from build123d import *

# Parameters (mm, degrees)
SKETCH1_W                = 19
SKETCH1_H                = 19
BOSS_EXTRUDE1_DEPTH      = 1.5
SKETCH2_W                = 5
SKETCH2_H                = 5
CUT_EXTRUDE1_DEPTH       = 30.054329533
BOSS_EXTRUDE2_DEPTH      = 10
BOSS_EXTRUDE2_DEPTH_BACK = 1.5
SKETCH4_W                = 1
SKETCH4_H                = 19
SKETCH5_W                = 21
SKETCH5_H                = 1
BOSS_EXTRUDE3_DEPTH      = 19
SKETCH6_W                = 5
SKETCH6_H                = 5
CUT_EXTRUDE2_DEPTH       = 33.074717791
SKETCH7_W                = 3.862532253
SKETCH7_H                = 19
CUT_EXTRUDE3_DEPTH       = 1


with BuildPart() as part:
    # Sketch1 → Boss-Extrude1 (new body)
    with BuildSketch(Plane.XY):
        with Locations((-17.316728365, -1.580033592)):
            Rectangle(SKETCH1_W, SKETCH1_H)
    extrude(amount=BOSS_EXTRUDE1_DEPTH)

    # Sketch2 → Cut-Extrude1 (cut, through all)
    with BuildSketch(Plane(origin=(0, 0, 0), x_dir=(-1, 0, 0), z_dir=(0, 0, -1))):
        with Locations((22.031286711, -1.437353134)):
            Rectangle(SKETCH2_W, SKETCH2_H)
    extrude(amount=-CUT_EXTRUDE1_DEPTH, mode=Mode.SUBTRACT)

    # Sketch4 → Boss-Extrude2 (add, two sides: drawn at the far end of the back side and taken through both)
    with BuildSketch(Plane.XY.offset(1.5).offset(-BOSS_EXTRUDE2_DEPTH_BACK)):
        with Locations((-7.316728365, -1.580033592)):
            Rectangle(SKETCH4_W, SKETCH4_H)
        with Locations((-27.316728365, -1.580033592)):
            Rectangle(SKETCH4_W, SKETCH4_H)
    extrude(amount=BOSS_EXTRUDE2_DEPTH + BOSS_EXTRUDE2_DEPTH_BACK)

    # Sketch5 → Boss-Extrude3 (add)
    with BuildSketch(Plane(origin=(0, 7.919966408, 0), x_dir=(-1, 0, 0), z_dir=(0, 1, 0))):
        with Locations((17.316728365, 12)):
            Rectangle(SKETCH5_W, SKETCH5_H)
    extrude(amount=-BOSS_EXTRUDE3_DEPTH)

    # Sketch6 → Cut-Extrude2 (cut, through all)
    with BuildSketch(Plane(origin=(0, 0, 11.5), x_dir=(-1, 0, 0), z_dir=(0, 0, -1))):
        with Locations((22.031286711, -1.437353134)):
            Rectangle(SKETCH6_W, SKETCH6_H)
    extrude(amount=-CUT_EXTRUDE2_DEPTH, mode=Mode.SUBTRACT)

    # Sketch7 → Cut-Extrude3 (cut)
    with BuildSketch(Plane(origin=(0, 0, 12.5), x_dir=(-1, 0, 0), z_dir=(0, 0, -1))):
        with Locations((15.385462239, -1.580033592)):
            Rectangle(SKETCH7_W, SKETCH7_H)
    extrude(amount=CUT_EXTRUDE3_DEPTH, mode=Mode.SUBTRACT)


solid = part.part
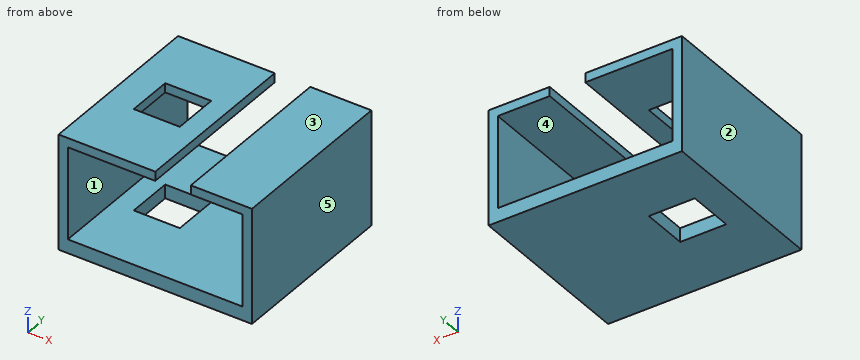
The model under review builds one solid part; all positions refer to its coordinate system, in mm. Face numbers are marked on the shaded views. A direction names the side the tool comes from. Give positions to 0.01 mm unless a question says otherwise; leave off trailing zeros. Order: outer loops, then holes, each group sorted by start corner. A loop starts at its lowest first (then second) coordinate and runs counter-clockwise, first axis right, second up. Notation, with made-up numbers: M 60,-2.75 L 76,-2.75 A27 ccw 76,24.25 Z; hole C -3,55 d4. An arc over 180 degrees is marked long. One line per question, with ' | ' between items. Start each with the question number.
1) Consider section C-C, the plane y = -2.5. Give the boundary of the cut face in (x, z), then the cut area to 3 significant figures.
2) For the marked faces 4 and 5, list the 3-axis set-ups (+Z, -Z, +X, -X, +Y, -Y) from which the entire face can be reached by the end or side of a thin tool; tool diameter is ignored.
3) Mouldability with a two-part tool opening along Z and no side actions: class the marked faces 1, 2 and 3 as pulls with the +Z half, pulls with the -Z half, needs draft (parallel to the pull), parting line crosses it, or undercut.
4) Wall thickness on L1, parallel to X at y = -6, z = 12.25; L2, parallel to Z at x = -23.5, y = 5; L3, parallel to X at y = 4.5, z = 2.5: over which ranges is each line inside the solid? List them lowest first. Write a range as from..to.
5) Consider section B-B, the plane x = -23.75. Give the boundary of the cut face in (y, z).
6) Consider section A-A, the plane z = 9.5. Give the boundary of the cut face in (x, y).
7) Consider section D-D, the plane x = -19. Give the boundary of the cut face in (y, z).
Found:
1) outline: M -27.82,0 L -24.53,0 L -24.53,1.5 L -26.82,1.5 L -26.82,11.5 L -24.53,11.5 L -24.53,12.5 L -27.82,12.5 Z; M -19.53,0 L -6.82,0 L -6.82,12.5 L -13.45,12.5 L -13.45,11.5 L -7.82,11.5 L -7.82,1.5 L -19.53,1.5 Z; M -19.53,11.5 L -17.32,11.5 L -17.32,12.5 L -19.53,12.5 Z | area: 56.1 mm²
2) face 4: +Y, -Y | face 5: +Z, -Z, +X, +Y, -Y
3) face 1: undercut | face 2: needs draft | face 3: pulls with the +Z half
4) L1: x = -27.82..-17.32, -13.45..-6.82 | L2: z = 0..1.5, 11.5..12.5 | L3: x = -27.82..-26.82, -7.82..-6.82
5) outline: M -11.08,0 L -3.94,0 L -3.94,1.5 L -11.08,1.5 Z; M -11.08,11.5 L -3.94,11.5 L -3.94,12.5 L -11.08,12.5 Z; M 1.06,0 L 7.92,0 L 7.92,1.5 L 1.06,1.5 Z; M 1.06,11.5 L 7.92,11.5 L 7.92,12.5 L 1.06,12.5 Z
6) outline: M -27.82,-11.08 L -26.82,-11.08 L -26.82,7.92 L -27.82,7.92 Z; M -7.82,-11.08 L -6.82,-11.08 L -6.82,7.92 L -7.82,7.92 Z
7) outline: M -11.08,0 L 7.92,0 L 7.92,1.5 L -11.08,1.5 Z; M -11.08,11.5 L 7.92,11.5 L 7.92,12.5 L -11.08,12.5 Z
